Autodesk Inventor part; units mm, degrees
ref_plane "YZ Plane" through (0, 0, 0) normal (1, 0, 0) x (0, 1, 0)
ref_plane "XZ Plane" through (0, 0, 0) normal (0, 1, 0) x (-1, 0, 0)
ref_plane "XY Plane" through (0, 0, 0) normal (0, 0, 1) x (1, 0, 0)
sketch "Sketch1" plane through (0, 0, 0) normal (0, 1, 0) x (-1, 0, 0)
  line L0 (825, 12.5) -> (-825, 12.5)
  line L1 (-825, 12.5) -> (-825, -12.5)
  line L2 (-825, -12.5) -> (825, -12.5)
  line L3 (825, -12.5) -> (825, 12.5)
  line L4 (825, 12.5) -> (-825, -12.5) construction
  line L5 (-825, 12.5) -> (825, -12.5) construction
  point P0 (0, 0)
  dimension "d0" = 1650
  dimension "d1" = 25
extrude "Plate1" add sketch "Sketch1" along normal blind 3.2
sketch "Sketch2" plane through (825, 0, 9.3) normal (0, 0, 1) x (1, 0, 0)
  line L0 (-1650, 0) -> (0, 0)
  line L1 (0, 0) -> (0, 25)
  line L2 (0, 25) -> (-1650, 25)
  line L3 (-1650, 25) -> (-1650, 0)
edge flange "Flange1" height 25 angle 90 thickness 3.2 bend radius 1.516 thickness toward (0, 0, 1) relief tear relief width 3.2 relief depth 1.6 edges at (0, 3.2, 12.5) wall of the first edge with corners at (-825, 0, 9.3) (825, 0, 9.3) (825, 25, 9.3) (-825, 25, 9.3)
bend "Bend1"
corner "Corner1"
sketch "Sketch3" plane through (825, 25, 9.3) normal (0, 0, -1) x (-1, 0, 0)
  circle A0 centre (105, -10.45) radius 1.5706
  circle A1 centre (285, -10.45) radius 1.5706
  circle A2 centre (465, -10.45) radius 1.5706
  circle A3 centre (825, -10.45) radius 1.5706
  circle A4 centre (1005, -10.45) radius 1.5706
  circle A5 centre (1185, -10.45) radius 1.5706
  circle A6 centre (1365, -10.45) radius 1.5706
  circle A7 centre (1545, -10.45) radius 1.5706
  point P0 (825, -25)
hole "Hole1" at (540, 14.55, 9.3) at (720, 14.55, 9.3) at (360, 14.55, 9.3) at (0, 14.55, 9.3) at (-180, 14.55, 9.3) at (-360, 14.55, 9.3) at (-540, 14.55, 9.3) at (-720, 14.55, 9.3) direction (0, 0, 1) diameter 4.5 depth 3.2 tip angle 118
sketch "Sketch8" plane through (0, 0, 0) normal (0, -1, 0) x (1, 0, 0)
  line L0 (-825, -12.5) -> (825, -12.5)
  line L1 (0, -12.5) -> (0, -2.5)
  line L2 (0, -2.5) -> (-270, -2.5)
  line L3 (-270, -2.5) -> (-790, -2.5)
  line L4 (0, -2.5) -> (270, -2.5)
  line L5 (270, -2.5) -> (790, -2.5)
  point P0 (0, 0)
  dimension "d40" = 10
  dimension "d41" = 270
  dimension "d42" = 520
  dimension "d43" = 180
hole "Hole2" at (-790, 0, -2.5) at (-270, 0, -2.5) at (270, 0, -2.5) at (790, 0, -2.5) direction (0, 1, 0) diameter 4.5 depth 3.2 tip angle 118
fillet "Corner Round1" radius 3 4 edges at (825, 1.6, -12.5) (-825, 25, 10.9) (825, 25, 10.9) (-825, 1.6, -12.5)
equation "\"d18\" = Thickness"
equation "\"d37\" = Thickness"
equation "\"d2\" = Thickness"
equation "\"d3\" = BendReliefWidth"
equation "\"d4\" = BendReliefDepth"
equation "\"d5\" = MinimumRemnant"
equation "\"d6\" = TransitionRadius"
equation "\"d9\" = BendRadius"
equation "\"d10\" = CornerReliefSize"
equation "\"d11\" = GapSize"
equation "\"d12\" = JacobiRadiusSize"
equation "\"BendReliefWidth\" = Thickness"
equation "\"BendReliefDepth\" = 0.5 * Thickness"
equation "\"CornerReliefSize\" = 4 * Thickness"
equation "\"MinimumRemnant\" = 2 * Thickness"
equation "\"TransitionRadius\" = BendRadius"
equation "\"JacobiRadiusSize\" = BendRadius"
equation "\"GapSize\" = Thickness"
properties part number "SP39V1 Chapa Acrilico" material "Steel, Carbon"
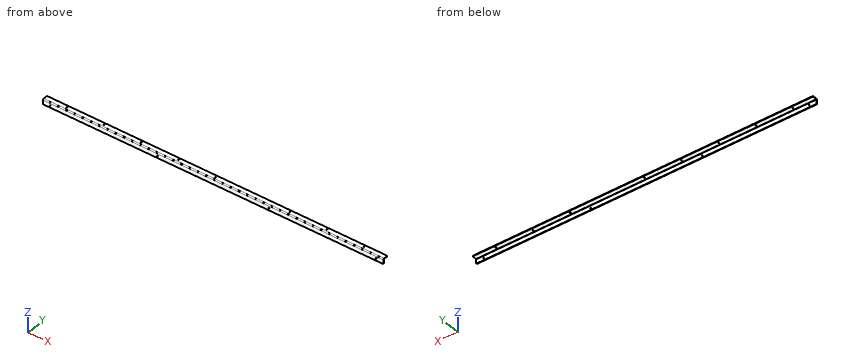
The listing builds one solid part. Answer for the finished solid, in the listing's coordinates (mm). Round coordinates to 2 decimals unless told otherwise and drop trailing zeros. Order: outer loops, then holes, each group sorted by start corner. A loop starts at its lowest first (then second) coordinate and runs counter-clockwise, first axis right, second up. Notation, with made-up numbers: M 43.5,77 L 102.5,77 A9 cw 102.5,90 Z; hole C 25.25,-39 d6. An arc over 180 degrees is marked long. Answer in a Markdown table with one row per item. Add a question column.
1) Flat-ended cylindrical pins translate along their axes: pin 1 Ø5 at (x, y) = (-720, 14.55) entering from +Z; pin 2 Ø7 at (x, y) = (360, 14.55) entering from -Z; pin 3 Ø5 at (x, z) = (-790, -2.5) entering from +Y. Find the tip coordinate at first contact, or state that the pin passes through.
2) The part is cut by section A-A on x = 608. Determine the outline of the cut face in (y, z).
3) Consider line 1 along X through (y, z) = (1.1, -2.5); line 2 along Z through (x, y) = (346.5, 5.75); line 3 along Y through (x, z) = (-219, -9). Determine where each line is inside the solid, lowest interval first. Write a range as from..to.
Findings below:
| question | item | result |
|---|---|---|
| 1 | pin 1 | stops at z = 12.5 |
| 1 | pin 2 | stops at z = 9.3 |
| 1 | pin 3 | stops at y = 3.2 |
| 2 | outline | M 0,-12.5 L 3.2,-12.5 L 3.2,7.78 A1.52 cw 4.72,9.3 L 25,9.3 L 25,12.5 L 4.72,12.5 A4.72 ccw 0,7.78 Z |
| 3 | line 1 | x = -825..-792.25, -787.75..-272.25, -267.75..267.75, 272.25..787.75, 792.25..825 |
| 3 | line 2 | z = 9.3..12.5 |
| 3 | line 3 | y = 0..3.2 |
